from build123d import *

# Parameters (mm, degrees)
F0_W     = 53.390044
F0_H     = 19.768442
F0_R     = 5
F1_DEPTH = 15
F3_W     = 53.390044
F3_H     = 33.533428
F4_DEPTH = 17.5
F5_R     = 2
F6_R     = 15
F2_R     = 5
F7_DEPTH = 44.269914


with BuildPart() as f1:
    # F0 (on Top) → F1 (new body)
    with BuildSketch(Plane.XY):
        Rectangle(F0_W, F0_H)
        with Locations((-18, 0)):
            Circle(F0_R, mode=Mode.SUBTRACT)
        with Locations((-6, 0)):
            Circle(F0_R, mode=Mode.SUBTRACT)
        with Locations((6, 0)):
            Circle(F0_R, mode=Mode.SUBTRACT)
        with Locations((18, 0)):
            Circle(F0_R, mode=Mode.SUBTRACT)
    extrude(amount=F1_DEPTH)

    # F3 (on face) → F4 (join)
    with BuildSketch(Plane(origin=(0, 0, 0), x_dir=(1, 0, 0), z_dir=(0, 0, -1))):
        Rectangle(F3_W, F3_H)
    extrude(amount=F4_DEPTH)

    # F5
    f5_edges = [f1.edges().sort_by_distance(p)[0] for p in [
        (0, 9.884221, 0),
        (0, -9.884221, 0),
    ]]
    fillet(f5_edges, radius=F5_R)

    # F6
    f6_edges = [f1.edges().sort_by_distance(p)[0] for p in [
        (0, -16.766714, 0),
        (0, 16.766714, 0),
    ]]
    fillet(f6_edges, radius=F6_R)

    # F2 (on face) → F7 (cut)
    with BuildSketch(Plane.XY.offset(15)):
        with Locations((-18, 0)):
            Circle(F2_R)
        with Locations((-6, 0)):
            Circle(F2_R)
        with Locations((6, 0)):
            Circle(F2_R)
        with Locations((18, 0)):
            Circle(F2_R)
    extrude(amount=-F7_DEPTH, mode=Mode.SUBTRACT)

    # F8 (on face) → F9 (revolve, cut)
    with BuildSketch(Plane(origin=(0, 0, -17.5), x_dir=(1, 0, 0), z_dir=(0, 0, -1))):
        with BuildLine():
            Line((26.695022, 0), (23, 0))
            ThreePointArc((23, 0), (18, -5), (13, 0))
            Line((13, 0), (11, 0))
            ThreePointArc((11, 0), (6, -5), (1, 0))
            Line((1, 0), (-1, 0))
            ThreePointArc((-1, 0), (-6, -5), (-11, 0))
            Line((-11, 0), (-13, 0))
            ThreePointArc((-13, 0), (-18, -5), (-23, 0))
            Line((-23, 0), (-26.695022, 0))
            Line((-26.695022, 0), (-26.695022, -3.5))
            Line((-26.695022, -3.5), (-25.195022, -3.5))
            Line((-25.195022, -3.5), (-25.195022, -14.766714))
            Line((-25.195022, -14.766714), (25.195022, -14.766714))
            Line((25.195022, -14.766714), (25.195022, -3.5))
            Line((25.195022, -3.5), (26.695022, -3.5))
            Line((26.695022, -3.5), (26.695022, 0))
        make_face()
    revolve(axis=Axis((0, 0, -17.5), (1, 0, 0)), mode=Mode.SUBTRACT)


solid = f1.part
Geometry check sheet. Reference: the model listing, model coordinates, mm. A direction names the side the tool comes from. Coordinates: 2 decimals unless noted, no trailing zeros. Write each loop counter-clockwise with the first axis right and the second up, starting at its lowest first coordinate (ties: lowest second). Pieces come first, ordered by that corner, then holes. Notation, with made-up numbers: (67, 83) -> (88, 83) arc R34 cw to (88, 113) -> close; hole circle Ø4 at (74.25, -31.75). An arc over 180 degrees is marked (long way). One line per question, with ' | ' between items.
1. Cross-section at B-B on z = 3. Record the cut outline in (x, y).
Answers:
outline: (-26.7, -9.88) -> (26.7, -9.88) -> (26.7, 9.88) -> (-26.7, 9.88) -> close; hole circle Ø10 at (-18, 0); hole circle Ø10 at (-6, 0); hole circle Ø10 at (6, 0); hole circle Ø10 at (18, 0)
2. Thickness scan on probe 1 along X at (y, z) = (0, -1.6); probe 2 along Y at (x, z) = (6, 5.25); probe 3 along X at (y, z) = (3.5, -6). Record the ranges inside material, lowest first. Write a range as from..to.
Answers:
probe 1: x = -26.7..-23, -13..-11, -1..1, 11..13, 23..26.7 | probe 2: y = -9.88..-5, 5..9.88 | probe 3: x = -26.7..-25.2, 25.2..26.7
3. Cross-section at A-A on y = 0. Record the cut outline in (x, z).
Answers:
outline: (-26.7, -14) -> (-25.2, -14) -> (-25.2, -2.73) -> (-23, -2.73) -> (-23, 15) -> (-26.7, 15) -> close; (-13, -2.73) -> (-11, -2.73) -> (-11, 15) -> (-13, 15) -> close; (-1, -2.73) -> (1, -2.73) -> (1, 15) -> (-1, 15) -> close; (11, -2.73) -> (13, -2.73) -> (13, 15) -> (11, 15) -> close; (23, -2.73) -> (25.2, -2.73) -> (25.2, -14) -> (26.7, -14) -> (26.7, 15) -> (23, 15) -> close
4. Depth check by flat-ended pin: pin 1 Ø3 at (x, y) = (-14, 7) entering from -Z (3 decimals); pin 2 Ø2 at (x, z) = (9.5, 2) entering from -Y; pin 3 Ø5 at (x, y) = (-12, 6.5) entering from -Z; pin 4 Ø11.5 at (x, y) = (-18, 0) entering from +Z. Enter the tip coordinate at first touch or a pass-through.
Answers:
pin 1: stops at z = -5.425 | pin 2: stops at y = -10.15 | pin 3: stops at z = -5.79 | pin 4: stops at z = 15
5. Draft check along Y on faces 4 (the flat face through (26.695, 0, -5)), 5 (the cylindrical face through (0.4, -10.1, 1.1)), 6 (the cylindrical face through (26, 0, -14)), 7 (the cylindrical face through (0.4, 10.1, 1.1)). Enter one of: +Y half, -Y half, draft (parallel to the pull), parting line (faces both ways), or undercut.
Answers:
face 4: draft | face 5: -Y half | face 6: undercut | face 7: +Y half
6. Cross-section at C-C on z = -12.5. Record the cut outline in (x, y).
Answers:
outline: (-26.7, -16.77) -> (26.7, -16.77) -> (26.7, 16.77) -> (-26.7, 16.77) -> close; hole (-25.2, -13.89) -> (25.2, -13.89) -> (25.2, 13.89) -> (-25.2, 13.89) -> close
7. Set-up check for faces 1 (the flat face through (25.195, 0, -10)), 2 (the flat face through (0, 9.884, 8)), 3 (the flat face through (0, -9.884, 8)): record each of +Z, -Z, +X, -X, +Y, -Y from which the full face is reachable in a straight line by a thin tool's end or side.
Answers:
face 1: -Z | face 2: +Z, +X, -X, +Y | face 3: +Z, +X, -X, -Y
